Can you work these out from the drawing? Everything is in mm from the part's minimum corner. Round coordinates to 2 decimals unless told otherwise and drop trailing zeros. Loops run counter-clockwise (first coordinate to the right, second up) from the corner with the lowest first, then second, coordinate; pieces in that order, holes last. Notation, with made-up numbers: (87.25, 52.25) -> (107.25, 52.25) arc R16 ccw to (107.25, 62.25) -> close; hole circle Ø2 at (72, -15). An arc over 180 degrees is marked (long way). One line per item, written item: value.
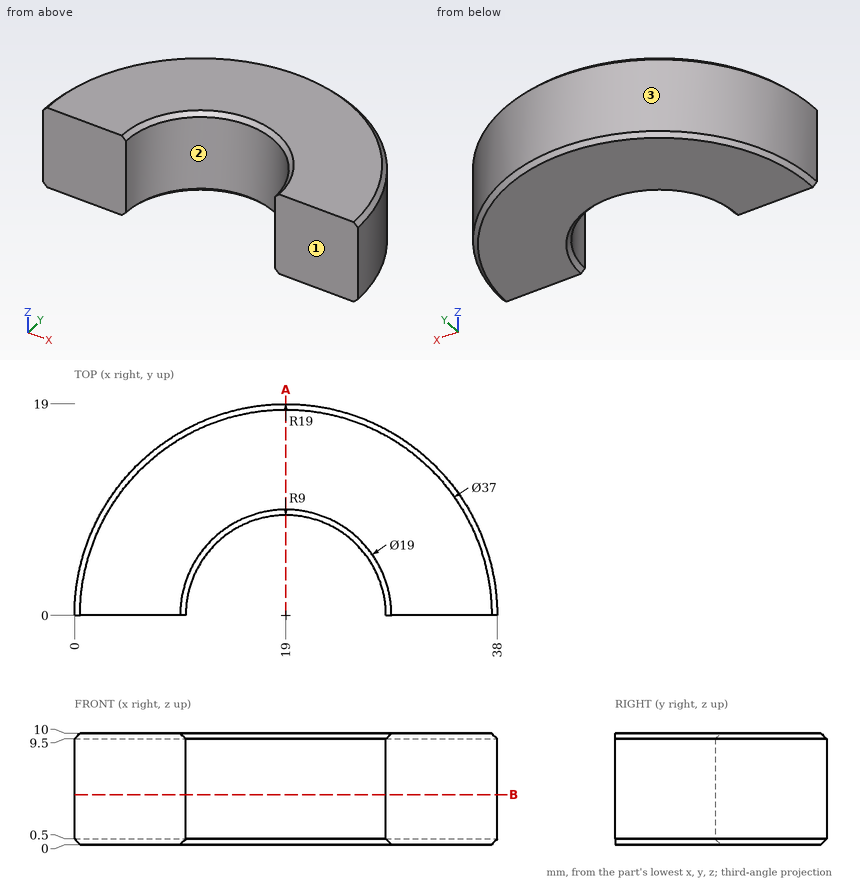
(1) I'm going to push flat-ended pins straight in: pin 1 Ø6 at (y, z) = (5.5, 6) entering from +X; pin 2 Ø2 at (x, z) = (21, 3) entering from -Y; pin 3 Ø5 at (y, z) = (10, 2.5) entering from +X. Where does each tip first touch, or does it pass through?
Recorded:
pin 1: x = 37.83
pin 2: y = 8.49
pin 3: x = 36.46
(2) If we section it at A-A, the plane x = 19: Please give me the cut outline in (y, z), then the cut area to 3 significant figures.
Recorded:
outline: (9, 0.5) -> (9.5, 0) -> (18.5, 0) -> (19, 0.5) -> (19, 9.5) -> (18.5, 10) -> (9.5, 10) -> (9, 9.5) -> close
area: 99.5 mm²
(3) Thinking about a two-plate mould opening in X: for the marked faces 1, 2 and 3, which applies, released by +X, released by -X, zero draft, split by the parting line, or undercut?
Recorded:
face 1: zero draft
face 2: undercut
face 3: split by the parting line
(4) If we section it at B-B, the plane z = 4.5: Please give me the cut outline in (x, y), then the cut area to 3 significant figures.
Recorded:
outline: (0, 0) -> (10, 0) arc R9 cw to (28, 0) -> (38, 0) arc R19 ccw to start
area: 440 mm²
(5) If I drill on L1, parallel to X at y = 2, z = 2.75; L2, parallel to X at y = 7, z = 3.75; L3, parallel to Y at x = 2, z = 7, over which ranges is the centre line in solid material (lowest first)?
Recorded:
L1: 0.11 to 10.23, 27.77 to 37.89
L2: 1.34 to 13.34, 24.66 to 36.66
L3: 0 to 8.49
